from build123d import *

# Parameters (mm, degrees)
CROQUIS1_W                 = 26
CROQUIS1_H                 = 21
SALIENTE_EXTRUIR1_DEPTH    = 6
CORTAR_EXTRUIR1_DEPTH      = 26.416530054
CORTAR_EXTRUIR1_DEPTH_BACK = 26.416530054
CROQUIS2_R                 = 1.75
CROQUIS3_R                 = 0.875
CORTAR_EXTRUIR2_DEPTH      = 15
REDONDEO1_R                = 1
CHAFL_N1_SIZE              = 0.8
CHAFL_N2_SIZE              = 0.8
CORTAR_EXTRUIR3_DEPTH      = 3.4
CROQUIS5_R                 = 1.7
CORTAR_EXTRUIR4_DEPTH      = 40


with BuildPart() as part:
    # Croquis1 → Saliente-Extruir1 (new, symmetric)
    with BuildSketch(Plane.XY):
        Rectangle(CROQUIS1_W, CROQUIS1_H)
    extrude(amount=SALIENTE_EXTRUIR1_DEPTH, both=True)

    # Croquis2 → Cortar-Extruir1 (cut, two sides: drawn at the far end of the back side and taken through both)
    with BuildSketch(Plane.XZ.offset(10.5).offset(-CORTAR_EXTRUIR1_DEPTH_BACK)):
        with Locations(Location((-9, 0, 0), (0, 0, 270))):
            Circle(CROQUIS2_R)
        with Locations(Location((9, 0, 0), (0, 0, 270))):
            Circle(CROQUIS2_R)
    extrude(amount=CORTAR_EXTRUIR1_DEPTH + CORTAR_EXTRUIR1_DEPTH_BACK, mode=Mode.SUBTRACT)

    # Croquis3 → Cortar-Extruir2 (cut)
    with BuildSketch(Plane.XY.offset(6)):
        Circle(CROQUIS3_R)
    extrude(amount=-CORTAR_EXTRUIR2_DEPTH, mode=Mode.SUBTRACT)

    # Redondeo1
    redondeo1_edges = [part.edges().sort_by_distance(p)[0] for p in [
        (13, -10.5, 0),
        (-13, -10.5, 0),
        (-13, 10.5, 0),
        (13, 10.5, 0),
    ]]
    fillet(redondeo1_edges, radius=REDONDEO1_R)

    # Chaflán1
    chafl_n1_edges = [part.edges().sort_by_distance(p)[0] for p in [
        (0, 10.5, -6),
        (0, 10.5, 6),
        (13, 0, -6),
        (0, -10.5, -6),
        (-13, 0, -6),
        (-12.707106781, -10.207106781, -6),
        (12.707106781, -10.207106781, -6),
        (-12.707106781, 10.207106781, -6),
        (12.707106781, 10.207106781, -6),
        (13, 0, 6),
        (-13, 0, 6),
        (0, -10.5, 6),
        (-12.707106781, -10.207106781, 6),
        (12.707106781, -10.207106781, 6),
        (-12.707106781, 10.207106781, 6),
        (12.707106781, 10.207106781, 6),
    ]]
    chamfer(chafl_n1_edges, length=CHAFL_N1_SIZE)

    # Chaflán2
    chafl_n2_edges = [part.edges().sort_by_distance(p)[0] for p in [
        (-0.875, 0, -6),
        (-0.875, 0, 6),
    ]]
    chamfer(chafl_n2_edges, length=CHAFL_N2_SIZE)

    # Croquis4 → Cortar-Extruir3 (cut)
    with BuildSketch(Plane.XY.offset(6)):
        Polygon((-5.35, 3.0022214), (-7.95, 1.5011107), (-7.95, -1.5011107), (-5.35, -3.0022214), (-2.75, -1.5011107), (-2.75, 1.5011107), align=None)
        Polygon((5.35, 3.0022214), (2.75, 1.5011107), (2.75, -1.5011107), (5.35, -3.0022214), (7.95, -1.5011107), (7.95, 1.5011107), align=None)
    extrude(amount=-CORTAR_EXTRUIR3_DEPTH, mode=Mode.SUBTRACT)

    # Croquis5 → Cortar-Extruir4 (cut)
    with BuildSketch(Plane.XY.offset(2.6)):
        with Locations((5.35, 0)):
            Circle(CROQUIS5_R)
        with Locations((-5.35, 0)):
            Circle(CROQUIS5_R)
    extrude(amount=-CORTAR_EXTRUIR4_DEPTH, mode=Mode.SUBTRACT)


solid = part.part
Build history of the part. All positions in model axes, mm. A direction names the side the tool comes from. Coordinates: 2 decimals unless noted, no trailing zeros. Order: outer loops, then holes, each group sorted by start corner. A loop starts at its lowest first (then second) coordinate and runs counter-clockwise, first axis right, second up. Notation, with made-up numbers: (42, 30) - (58, 30) arc R30 ccw to (58, 69) - close; hole circle Ø7 at (-14, 50.5). An arc over 180 degrees is marked (long way). Write each question's results on one line, items separated by ' | '. Start each with the question number.
Item 1: Flat gauge pins, fed straight in: pin 1 (2.5 mm diameter, centred on x = 0, y = 0, fed in from +Z) (3 decimals); pin 2 (1.6 mm diameter, centred on x = 6, y = -1.5, fed in from +Z). Where does each tip first touch, or does it go through?
Item 2: Band-saw the part on D-D on z = 3.5. Write the cut outline in (x, y) (3 decimals).
Item 3: Wall check: probe 1 along Y at (x, z) = (5.25, -0.75); probe 2 along Z at (x, y) = (9, -5.75); probe 3 along X at (y, z) = (-3, -0.25). Give the ranges that are in metal, low to high. Write a range as [from, to].
Item 4: Tool access for faces 4 (the face through (-7.265, 0.147, 0.228)), 5 (the face through (6.632, -2.262, 4.324)): list every direction of +Z, -Z, +X, -X, +Y, -Y with a clear straight run to the whole face (end or side of a thin tool).
Item 5: Band-saw the part on C-C on z = -0.5. Write the cut outline in (x, y) (3 decimals).
Item 6: Band-saw the part on B-B on x = -9. Write the cut outline in (y, z), and give its area (3 significant figures).
Item 7: Mould opens along Y. For faces 1 (the face through (-12.433, 9.923, -5.594)), 2 (the face through (12.6, 0.1, 5.6)), 3 (the face through (6.67, 2.24, 4.32)) say: released by +Y, released by -Y, zero draft, split by the parting line, or undercut.
Item 8: Band-saw the part on A-A on y = 0. State how many separate pieces and enclosed holes the cut face has, and give its area (3 significant figures).
Numbers:
1) pin 1: z = 5.575 | pin 2: z = 2.6
2) outline: (-13, -9.5) arc R1 ccw to (-12, -10.5) - (12, -10.5) arc R1 ccw to (13, -9.5) - (13, 9.5) arc R1 ccw to (12, 10.5) - (-12, 10.5) arc R1 ccw to (-13, 9.5) - close; hole (-7.95, -1.501) - (-5.35, -3.002) - (-2.75, -1.501) - (-2.75, 1.501) - (-5.35, 3.002) - (-7.95, 1.501) - close; hole circle Ø1.75 at (0, 0); hole (2.75, -1.501) - (5.35, -3.002) - (7.95, -1.501) - (7.95, 1.501) - (5.35, 3.002) - (2.75, 1.501) - close
3) probe 1: [-10.5, -1.7], [1.7, 10.5] | probe 2: [-6, -1.75], [1.75, 6] | probe 3: [-13, -10.73], [-7.27, 7.27], [10.73, 13]
4) face 4: +Y, -Y | face 5: +Z
5) outline: (-13, -9.5) arc R1 ccw to (-12, -10.5) - (-10.677, -10.5) - (-10.677, 10.5) - (-12, 10.5) arc R1 ccw to (-13, 9.5) - close; (-7.323, -10.5) - (7.323, -10.5) - (7.323, 10.5) - (-7.323, 10.5) - close; (10.677, -10.5) - (12, -10.5) arc R1 ccw to (13, -9.5) - (13, 9.5) arc R1 ccw to (12, 10.5) - (10.677, 10.5) - close; hole circle Ø3.4 at (-5.35, 0); hole circle Ø1.75 at (0, 0); hole circle Ø3.4 at (5.35, 0)
6) outline: (-10.5, -5.2) - (-9.7, -6) - (9.7, -6) - (10.5, -5.2) - (10.5, -1.75) - (-10.5, -1.75) - close; (-10.5, 1.75) - (10.5, 1.75) - (10.5, 5.2) - (9.7, 6) - (-9.7, 6) - (-10.5, 5.2) - close | area: 177 mm^2
7) face 1: released by +Y | face 2: zero draft | face 3: undercut
8) separate pieces: 4 | enclosed holes: 2 | area: 175 mm^2
